Design review of the part shown in the three views and the two pictorial views. Dimensions are in mm from the part's minimum x, y and z. Coordinates: 2 decimals unless noted, no trailing zeros. Write each loop counter-clockwise with the first axis right and the second up, starting at its lowest first coordinate (ties: lowest second). Pieces come first, ordered by that corner, then holes. Notation, with made-up numbers: M 23.25,35 L 41.25,35 A16 cw 41.25,53 Z; hole C 48.5,-14 d9. An arc over 180 degrees is marked long. One line per question, with ' | ' between items.
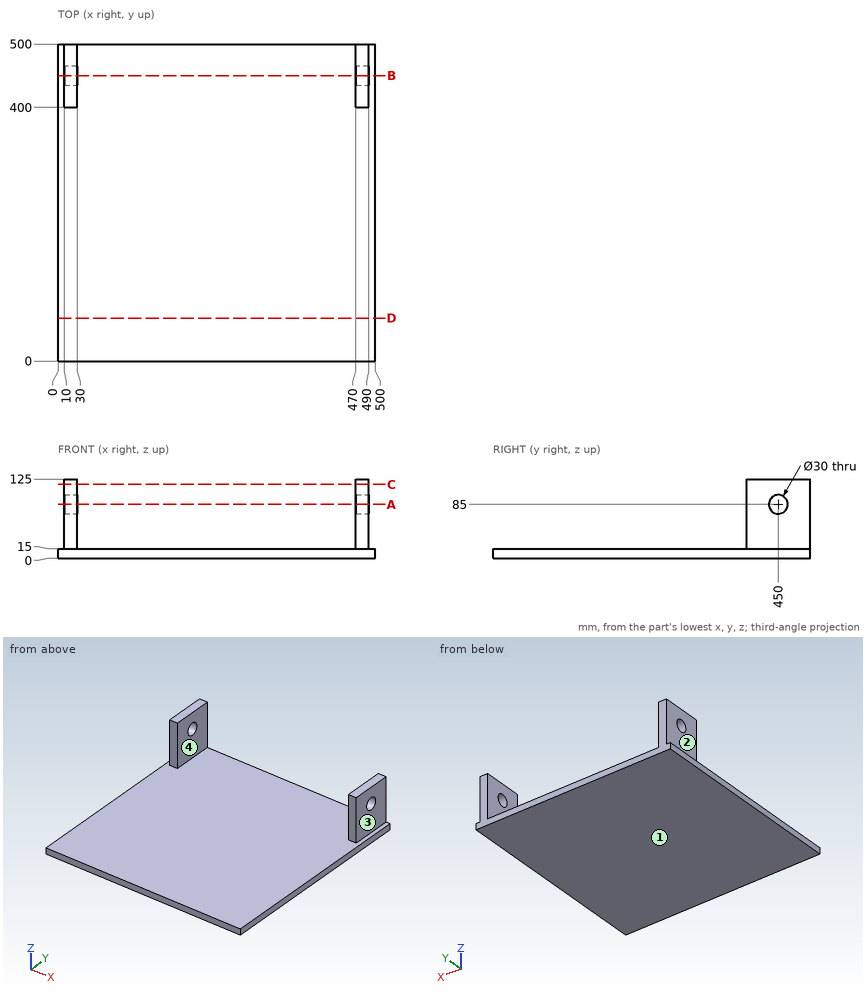
1. Take a section at A-A on z = 85. State the section outline as (x, y) points, plus the area to 3 significant figures.
Computed values:
outline: M 10,400 L 30,400 L 30,435 L 10,435 Z; M 10,465 L 30,465 L 30,500 L 10,500 Z; M 470,400 L 490,400 L 490,435 L 470,435 Z; M 470,465 L 490,465 L 490,500 L 470,500 Z | area: 2,800 mm2
2. Take a section at C-C on z = 116.5. State the section outline as (x, y) points.
Computed values:
outline: M 10,400 L 30,400 L 30,500 L 10,500 Z; M 470,400 L 490,400 L 490,500 L 470,500 Z
3. Draft analysis for pull direction X (two halves, no side actions). For the marked faces 1, 2, 3 and 4, state which applies: pulls with the +X half, pulls with the -X half, needs draft (parallel to the pull), parting line crosses it, or undercut.
Computed values:
face 1: needs draft | face 2: pulls with the -X half | face 3: pulls with the +X half | face 4: undercut
4. Take a section at D-D on y = 67.5. State the section outline as (x, z) points.
Computed values:
outline: M 0,0 L 500,0 L 500,15 L 0,15 Z
5. Clearance check with flat-ended pins moving along their axes: P1, Ø16, axis at x = 21.5, z = 80.5, coming from the -Y side; P2, Ø4, axis at x = 50.5, y = 407.5, coming from the +Z side. State where each tip first meets the part, or that it passes through.
Computed values:
P1: stops at y = 400 | P2: stops at z = 15
6. Take a section at B-B on y = 450. State the section outline as (x, z) points.
Computed values:
outline: M 0,0 L 500,0 L 500,15 L 490,15 L 490,70 L 470,70 L 470,15 L 30,15 L 30,70 L 10,70 L 10,15 L 0,15 Z; M 10,100 L 30,100 L 30,125 L 10,125 Z; M 470,100 L 490,100 L 490,125 L 470,125 Z
7. For line 1 along Z through (x, y) = (20, 450); line 2 along X through (y, z) = (429, 51); line 3 along Z through (x, y) = (462.5, 166), list the stretches that pass through material, from the lowest coordinate up.
Computed values:
line 1: z = 0 to 70, 100 to 125 | line 2: x = 10 to 30, 470 to 490 | line 3: z = 0 to 15
